from build123d import *

# Parameters (mm, degrees)
SKETCH1_W           = 86.7
SKETCH1_H           = 118.61
SKETCH1_W_2         = 14
SKETCH1_H_2         = 14
BOSS_EXTRUDE1_DEPTH = 1.5


# Read off the part's stored shape, not the designer's step: CSK for #0 Flat Head Machine Screw (100)1
with BuildPart() as part:
    # Sketch1 → Boss-Extrude1 (new body)
    with BuildSketch(Plane.XY):
        with Locations((-43.35, 59.305)):
            Rectangle(SKETCH1_W, SKETCH1_H)
        with Locations((-23.35, 37)):
            Rectangle(SKETCH1_W_2, SKETCH1_H_2, mode=Mode.SUBTRACT)
        with Locations((-23.35, 79)):
            Rectangle(SKETCH1_W_2, SKETCH1_H_2, mode=Mode.SUBTRACT)
        with Locations((-43.35, 79)):
            Rectangle(SKETCH1_W_2, SKETCH1_H_2, mode=Mode.SUBTRACT)
        with Locations((-63.35, 79)):
            Rectangle(SKETCH1_W_2, SKETCH1_H_2, mode=Mode.SUBTRACT)
        with Locations((-23.35, 59)):
            Rectangle(SKETCH1_W_2, SKETCH1_H_2, mode=Mode.SUBTRACT)
        with Locations((-43.35, 59)):
            Rectangle(SKETCH1_W_2, SKETCH1_H_2, mode=Mode.SUBTRACT)
        with Locations((-63.35, 59)):
            Rectangle(SKETCH1_W_2, SKETCH1_H_2, mode=Mode.SUBTRACT)
        with Locations((-43.35, 37)):
            Rectangle(SKETCH1_W_2, SKETCH1_H_2, mode=Mode.SUBTRACT)
        with Locations((-63.35, 37)):
            Rectangle(SKETCH1_W_2, SKETCH1_H_2, mode=Mode.SUBTRACT)
        with Locations((-33.35, 17)):
            Rectangle(SKETCH1_W_2, SKETCH1_H_2, mode=Mode.SUBTRACT)
        with Locations((-53.35, 17)):
            Rectangle(SKETCH1_W_2, SKETCH1_H_2, mode=Mode.SUBTRACT)
    extrude(amount=BOSS_EXTRUDE1_DEPTH)

    # CSK for _0 Flat Head Machine Screw _ 2 → CSK for #0 Flat Head Machine Screw (100)1 (revolve, cut)
    with BuildSketch(Plane(origin=(-5.08, 5.08, 0), x_dir=(1, 0, 0), z_dir=(0, -1, 0))):
        Polygon((0, 0), (1.778, 0), (1.778, 0.327777815), (3.175, 1.5), (0, 1.5), align=None)
    revolve(axis=Axis((-5.08, 5.08, 0), (0, 0, 1)), mode=Mode.SUBTRACT)

    # CSK for _0 Flat Head Machine Screw _ 3 o → CSK for _0 Flat Head Machine Screw _ 3 (revolve, cut)
    with BuildSketch(Plane(origin=(-81.62, 5.08, 0), x_dir=(1, 0, 0), z_dir=(0, -1, 0))):
        Polygon((0, 0), (1.778, 0), (1.778, 0.327777815), (3.175, 1.5), (0, 1.5), align=None)
    revolve(axis=Axis((-81.62, 5.08, 0), (0, 0, 1)), mode=Mode.SUBTRACT)

    # CSK for _0 Flat Head Machine Screw _ 4 o → CSK for _0 Flat Head Machine Screw _ 4 (revolve, cut)
    with BuildSketch(Plane(origin=(-81.62, 113.53, 0), x_dir=(1, 0, 0), z_dir=(0, -1, 0))):
        Polygon((0, 0), (1.778, 0), (1.778, 0.327777815), (3.175, 1.5), (0, 1.5), align=None)
    revolve(axis=Axis((-81.62, 113.53, 0), (0, 0, 1)), mode=Mode.SUBTRACT)

    # CSK for _0 Flat Head Machine Screw _ 5 o → CSK for _0 Flat Head Machine Screw _ 5 (revolve, cut)
    with BuildSketch(Plane(origin=(-5.08, 113.53, 0), x_dir=(1, 0, 0), z_dir=(0, -1, 0))):
        Polygon((0, 0), (1.778, 0), (1.778, 0.327777815), (3.175, 1.5), (0, 1.5), align=None)
    revolve(axis=Axis((-5.08, 113.53, 0), (0, 0, 1)), mode=Mode.SUBTRACT)


solid = part.part
Check sheet for the modelled part. Datum: model origin and axes. Units: mm. Round coordinates to 2 decimals unless told otherwise and drop trailing zeros. Loops run counter-clockwise (first coordinate to the right, second up) from the corner with the lowest first, then second, coordinate; pieces in that order, holes last. Notation, with made-up numbers: (-2.75, -17) -> (16.25, -17) arc R22 cw to (16.25, 21) -> close; hole circle Ø9 at (17.5, -38.5). An arc over 180 degrees is marked (long way). Put each result on its own line as item: value. Start each with the question number.
1. Scan lines: probe 1 along Y at (x, z) = (-5.08, 0.1); probe 2 along X at (y, z) = (84, 1.45); probe 3 along Y at (x, z) = (-69.5, 0.9). Record each from-to range of solid material in increasing order.
2. Section check C-C (x = -43). Enter the section's corners in (y, z), plus the area to 3 significant figures.
3. Gauge pin test, flat end, axial feed: pin 1 (2 mm diameter, centred on x = -81.62, y = 5.08, fed in from -Z). Record the tip position at first contact, or that the pin passes through.
4. Section check B-B (x = -81.62). Enter the section's corners in (y, z) (3 decimals).
5. Section check A-A (y = 5.08). Enter the section's corners in (x, z) (3 decimals).
6. Draft check along X on faces 1 (the face through (-82.005, 111.794, 0.166)), 2 (the face through (-34, 60, 0)). Enter one of: +X half, -X half, draft (parallel to the pull), parting line (faces both ways), or undercut.
7. Section check D-D (z = 0.75). Give the number of separate pieces and of enclosed holes in the cut face, plus the area to 3 significant figures.
Findings:
1. probe 1: y = 0 to 3.3, 6.86 to 111.75, 115.31 to 118.61
1. probe 2: x = -86.7 to -70.35, -56.35 to -50.35, -36.35 to -30.35, -16.35 to 0
1. probe 3: y = 0 to 30, 44 to 52, 66 to 72, 86 to 118.61
2. outline: (0, 0) -> (30, 0) -> (30, 1.5) -> (0, 1.5) -> close; (44, 0) -> (52, 0) -> (52, 1.5) -> (44, 1.5) -> close; (66, 0) -> (72, 0) -> (72, 1.5) -> (66, 1.5) -> close; (86, 0) -> (118.61, 0) -> (118.61, 1.5) -> (86, 1.5) -> close
2. area: 115 mm^2
3. pin 1: passes through
4. outline: (0, 0) -> (3.302, 0) -> (3.302, 0.328) -> (1.905, 1.5) -> (0, 1.5) -> close; (6.858, 0) -> (111.752, 0) -> (111.752, 0.328) -> (110.355, 1.5) -> (8.255, 1.5) -> (6.858, 0.328) -> close; (115.308, 0) -> (118.61, 0) -> (118.61, 1.5) -> (116.705, 1.5) -> (115.308, 0.328) -> close
5. outline: (-86.7, 0) -> (-83.398, 0) -> (-83.398, 0.328) -> (-84.795, 1.5) -> (-86.7, 1.5) -> close; (-79.842, 0) -> (-6.858, 0) -> (-6.858, 0.328) -> (-8.255, 1.5) -> (-78.445, 1.5) -> (-79.842, 0.328) -> close; (-3.302, 0) -> (0, 0) -> (0, 1.5) -> (-1.905, 1.5) -> (-3.302, 0.328) -> close
6. face 1: undercut
6. face 2: draft
7. separate pieces: 1
7. enclosed holes: 15
7. area: 8,060 mm^2
